Part model, mm, in its own coordinate system. A direction names the side the tool comes from. Round coordinates to 2 decimals unless told otherwise and drop trailing zeros. Loops run counter-clockwise (first coordinate to the right, second up) from the corner with the lowest first, then second, coordinate; pieces in that order, holes last.
1) Band-saw the part on C-C, the plane y = 35. Write the cut outline in (x, z).
2) Band-saw the part on B-B, the plane z = 25.5. Write the cut outline in (x, y).
3) Probe line 1 (Y direction, x = 30, z = 24); line 2 (X direction, y = 18.5, z = 17.5); line 3 (Z direction, x = 10.5, y = 24). List the from-to ranges inside material, lowest first.
4) Mould opens along Y. For faces 1 (the flat face through (47, 20, 23)), 2 (the flat face through (23, 0, 21)), 3 (the cylindrical face through (43.99, 38.15, 22.68)), 4 (the cylindrical face through (42.15, 35.99, 21.8)) say: +Y half, -Y half, draft (parallel to the pull), parting line (faces both ways), or undercut.
5) 3-axis set-ups, long thin cutter, end or side, ignore diameter. For faces 5 (the cylindrical face through (5.5, 4.07, 44.52)), 6 (the cylindrical face through (41.99, 2.85, 21.8)): which of +Z, -Z, +X, -X, +Y, -Y reach the whole face in a straight line?
6) Drop flat-ended pins along their axis: P1, Ø3.5, axis at x = 7, y = 35, coming from the -Z side; P2, Ø1.8, axis at x = 7, y = 4, coming from the +Z side (1 decimal). Give the stop position or say it passes through.
7) Band-saw the part on A-A, the plane x = 22.5. Write the cut outline in (y, z).
8) Band-saw the part on D-D, the plane x = 16. Write the cut outline in (y, z).
Autodesk Inventor part; units mm, degrees
ref_plane "YZ Plane" through (0, 0, 0) normal (1, 0, 0) x (0, 1, 0)
ref_plane "XZ Plane" through (0, 0, 0) normal (0, 1, 0) x (-1, 0, 0)
ref_plane "XY Plane" through (0, 0, 0) normal (0, 0, 1) x (1, 0, 0)
sketch "Sketch1" plane through (0, 0, 0) normal (0, 0, 1) x (1, 0, 0)
  line L0 (0, 0) -> (0, 39)
  line L1 (0, 39) -> (45, 39)
  line L2 (45, 39) -> (45, 0)
  line L3 (45, 0) -> (0, 0)
  line L4 (0, 39) -> (-2, 39) construction
  line L5 (-2, 39) -> (-2, 41) construction
  line L6 (-2, 41) -> (47, 41)
  line L7 (47, 41) -> (47, -2)
  line L8 (47, -2) -> (-2, -2)
  line L9 (-2, -2) -> (-2, 41)
  dimension "d0" = 39
  dimension "d1" = 45
  dimension "d2" = 2
  dimension "d3" = 2
  dimension "d4" = 49
  dimension "d5" = 43
  dimension "d6" = 49
extrude "Extrusion1" add sketch "Sketch1" along normal blind 43
sketch "Sketch2" plane through (0, 0, 43) normal (0, 0, 1) x (1, 0, 0)
  line L0 (-2, -2) -> (47, 41) construction
  line L1 (47, 41) -> (-2, 41)
  line L2 (47, 41) -> (-2, 41)
  line L3 (-2, 41) -> (22.5, 19.5) construction
  line L4 (-2, 41) -> (-2, -2)
  line L5 (-2, -2) -> (47, -2)
  line L6 (-2, -2) -> (47, -2)
  line L7 (47, -2) -> (47, 41)
  line L8 (-2, 41) -> (47, 41)
  circle A0 centre (22.5, 19.5) radius 5
  line L9 (27.5, 19.5) -> (40, 19.5) construction
  circle A1 centre (40, 19.5) radius 1.75
  point P0 (0, 0)
  dimension "d9" = 10
  dimension "d12" = 12.5
  dimension "d13" = 3.5
  dimension "d14" = 21.5
extrude "Extrusion3" add sketch "Sketch2" along normal blind 3
fillet "Fillet1" radius 10 8 edges at (-2, 41, 23) (0, 39, 21.5) (0, 0, 21.5) (-2, -2, 23) (47, -2, 23) (45, 0, 21.5) (47, 41, 23) (45, 39, 21.5)
chamfer "Chamfer1" distance 1 angle 45 1 edges at (38.25, 19.5, 46)
sketch "Sketch3" plane through (0, 0, 46) normal (0, 0, 1) x (1, 0, 0)
  circle A0 centre (22.5, 19.5) radius 5 construction
  line L0 (22.5, 19.5) -> (22.5, 41) construction
  line L1 (37, 41) -> (8, 41) construction
  line L2 (22.5, 19.5) -> (22.5, -2) construction
  line L3 (8, -2) -> (37, -2) construction
  line L4 (22.5, 19.5) -> (47, 19.5) construction
  line L5 (47, 19.5) -> (22.5, 19.5) construction
  line L6 (-2.181, 19.5) -> (22.5, 19.5) construction
  line L7 (38, 35) -> (38, 4) construction
  line L8 (38, 4) -> (7, 4) construction
  line L9 (7, 4) -> (7, 35) construction
  line L10 (7, 35) -> (38, 35) construction
  line L11 (38, 35) -> (7, 4) construction
  line L12 (38, 4) -> (7, 35) construction
  circle A1 centre (38, 35) radius 1.5
  circle A2 centre (7, 35) radius 1.5
  circle A3 centre (7, 4) radius 1.5
  circle A4 centre (38, 4) radius 1.5
  point P0 (0, 0)
  dimension "d22" = 31
  dimension "d23" = 31
  dimension "d24" = 3
  dimension "d25" = 3
  dimension "d26" = 3
  dimension "d27" = 3
extrude "Extrusion4" cut sketch "Sketch3" against normal blind 57.5
properties part number "Drill-NEMA17_Adapter"
Reported:
1. outline: (-1.17, 0) - (2, 0) - (2, 43) - (5.5, 43) - (5.5, 46) - (-1.17, 46) - close; (8.5, 43) - (36.5, 43) - (36.5, 46) - (8.5, 46) - close; (39.5, 43) - (43, 43) - (43, 0) - (46.17, 0) - (46.17, 46) - (39.5, 46) - close
2. outline: (-2, 8) arc R10 ccw to (8, -2) - (37, -2) arc R10 ccw to (47, 8) - (47, 31) arc R10 ccw to (37, 41) - (8, 41) arc R10 ccw to (-2, 31) - close; hole (0, 10) arc R10 ccw to (10, 0) - (35, 0) arc R10 ccw to (45, 10) - (45, 29) arc R10 ccw to (35, 39) - (10, 39) arc R10 ccw to (0, 29) - close
3. line 1: y = -2 to 0, 39 to 41
3. line 2: x = -2 to 0, 45 to 47
3. line 3: z = 43 to 46
4. face 1: draft
4. face 2: undercut
4. face 3: +Y half
4. face 4: undercut
5. face 5: +Z, -Z
5. face 6: -Z
6. P1: stops at z = 43
6. P2: passes through
7. outline: (-2, 0) - (0, 0) - (0, 43) - (14.5, 43) - (14.5, 46) - (-2, 46) - close; (24.5, 43) - (39, 43) - (39, 0) - (41, 0) - (41, 46) - (24.5, 46) - close
8. outline: (-2, 0) - (0, 0) - (0, 43) - (39, 43) - (39, 0) - (41, 0) - (41, 46) - (-2, 46) - close
